from build123d import *

# Parameters (mm, degrees)
SKETCH3_R               = 2
SKETCH3_R_2             = 2.5
BOSS_EXTRUDE3_DEPTH     = 10
SKETCH4_W               = 29.621982307
SKETCH4_H               = 15
SKETCH4_W_2             = 29.629902686
BOSS_EXTRUDE4_DEPTH     = 15
FILLET1_R               = 10
CUT_EXTRUDE1_DEPTH      = 57
CUT_EXTRUDE1_DEPTH_BACK = 15
SKETCH5_R               = 4
FILLET3_R               = 10


with BuildPart() as part:
    # Sketch3 → Boss-Extrude3 (new body)
    with BuildSketch(Plane(origin=(0, 0, 0), x_dir=(1, 0, 0), z_dir=(0, 1, 0))):
        with BuildLine():
            Line((-74.553080605, -18.028525235), (-74.553080605, 16.971474765))
            Line((-74.553080605, 16.971474765), (75.446919395, 16.971474765))
            Line((75.446919395, 16.971474765), (75.446919395, -18.028525235))
            Line((75.446919395, -18.028525235), (75.446919395, -59.351917417))
            ThreePointArc((75.446919395, -59.351917417), (72.517987207, -66.422985229), (65.446919395, -69.351917417))
            Line((65.446919395, -69.351917417), (49.960719272, -69.351917417))
            ThreePointArc((49.960719272, -69.351917417), (47.125982353, -68.941717551), (44.523807175, -67.744770737))
            Line((44.523807175, -67.744770737), (5.883831491, -42.713694512))
            ThreePointArc((5.883831491, -42.713694512), (0.446919395, -41.106547832), (-4.989992702, -42.713694512))
            Line((-4.989992702, -42.713694512), (-43.629968386, -67.744770737))
            ThreePointArc((-43.629968386, -67.744770737), (-46.232143563, -68.941717551), (-49.066880482, -69.351917417))
            Line((-49.066880482, -69.351917417), (-64.553080605, -69.351917417))
            ThreePointArc((-64.553080605, -69.351917417), (-71.624148417, -66.422985229), (-74.553080605, -59.351917417))
            Line((-74.553080605, -59.351917417), (-74.553080605, -18.028525235))
        make_face()
        with Locations(Location((-68.553080605, 11.471474765, 0), (0, 0, 270))):
            Circle(SKETCH3_R, mode=Mode.SUBTRACT)
        with Locations(Location((-50.553080605, 11.471474765, 0), (0, 0, 270))):
            Circle(SKETCH3_R, mode=Mode.SUBTRACT)
        with Locations(Location((-68.553080605, -12.528525235, 0), (0, 0, 270))):
            Circle(SKETCH3_R, mode=Mode.SUBTRACT)
        with Locations(Location((-50.553080605, -12.528525235, 0), (0, 0, 270))):
            Circle(SKETCH3_R, mode=Mode.SUBTRACT)
        with Locations(Location((51.446919395, -12.528525235, 0), (0, 0, 90))):
            Circle(SKETCH3_R, mode=Mode.SUBTRACT)
        with Locations(Location((69.446919395, -12.528525235, 0), (0, 0, 90))):
            Circle(SKETCH3_R, mode=Mode.SUBTRACT)
        with Locations(Location((69.446919395, 11.471474765, 0), (0, 0, 90))):
            Circle(SKETCH3_R, mode=Mode.SUBTRACT)
        with Locations(Location((51.446919395, 11.471474765, 0), (0, 0, 90))):
            Circle(SKETCH3_R, mode=Mode.SUBTRACT)
        with Locations(Location((-50.553080605, -47.693315976, 0), (0, 0, 270))):
            Circle(SKETCH3_R_2, mode=Mode.SUBTRACT)
        with Locations(Location((51.446919395, -47.693315976, 0), (0, 0, 90))):
            Circle(SKETCH3_R_2, mode=Mode.SUBTRACT)
    extrude(amount=BOSS_EXTRUDE3_DEPTH)

    # Sketch4 → Boss-Extrude4 (add)
    with BuildSketch(Plane.XZ):
        with Locations((-59.742089452, 0)):
            Rectangle(SKETCH4_W, SKETCH4_H)
        with Locations((60.624047673, 0)):
            Rectangle(SKETCH4_W_2, SKETCH4_H)
        with Locations((60.624047673, 51.713197214)):
            Rectangle(SKETCH4_W_2, SKETCH4_H)
        with Locations((-59.742089452, 51.713197214)):
            Rectangle(SKETCH4_W, SKETCH4_H)
    extrude(amount=BOSS_EXTRUDE4_DEPTH)

    # Fillet1
    fillet1_edges = [part.edges().sort_by_distance(p)[0] for p in [
        (-44.931098298, -15, 0),
        (-74.553080605, -15, 0),
        (75.438999016, -15, 0),
        (45.80909633, -15, 0),
    ]]
    fillet(fillet1_edges, radius=FILLET1_R)

    # Sketch5 → Cut-Extrude1 (cut, two sides: drawn at the far end of the back side and taken through both)
    with BuildSketch(Plane.XY.offset(7.5).offset(-CUT_EXTRUDE1_DEPTH_BACK)):
        with Locations(Location((-59.742089451, -7.004049179, 0), (0, 0, 180))):
            Circle(SKETCH5_R)
        with Locations(Location((60.620087484, -7.004049179, 0), (0, 0, 180))):
            Circle(SKETCH5_R)
    extrude(amount=CUT_EXTRUDE1_DEPTH + CUT_EXTRUDE1_DEPTH_BACK, mode=Mode.SUBTRACT)

    # Fillet3
    fillet3_edges = [part.edges().sort_by_distance(p)[0] for p in [
        (45.80909633, -15, 51.713197214),
        (75.438999016, -15, 51.713197214),
        (-74.553080605, -15, 51.713197214),
        (-44.931098298, -15, 51.713197214),
    ]]
    fillet(fillet3_edges, radius=FILLET3_R)


solid = part.part
For this review, take the finished solid that the model builds, in its own axes (mm). A direction names the side the tool comes from. Round coordinates to 2 decimals unless told otherwise and drop trailing zeros. Loops run counter-clockwise (first coordinate to the right, second up) from the corner with the lowest first, then second, coordinate; pieces in that order, holes last. Notation, with made-up numbers: (40.25, 8.5) - (59.25, 8.5) arc R29 cw to (59.25, 29.5) - close; hole circle Ø4 at (-25.75, 23). An arc over 180 degrees is marked (long way). Use one line per item in the form item = value.
1) Wall thickness on probe 1 along X at (y, z) = (-2.5, 50); probe 2 along Z at (x, y) = (48, -4); probe 3 along Z at (x, y) = (-67, 6.5): over which ranges is each line inside the solid? List them lowest first.
Solutions:
probe_1 = -74.55 to -44.93, 45.81 to 75.44
probe_2 = -7.5 to 7.5, 44.21 to 59.21
probe_3 = -16.97 to -12.73, -10.21 to 11.27, 13.79 to 69.05
2) Clearance check with flat-ended pins moving along their axes: P1, Ø7.5, axis at x = -59.5, y = -9.5, coming from the -Z side; P2, Ø2.5, axis at y = -3, z = -1.5, coming from the +X side; P3, Ø4.5, axis at x = -68.55, z = 12.53, coming from the -Y side; P4, Ø3.5, axis at x = -50.55, z = -11.47, coming from the -Y side. State where each tip first meets the part, or that it passes through.
Solutions:
P1 = -7.5
P2 = 75.44
P3 = 0
P4 = through
3) Mouldability with a two-part tool opening along Z and no side actions: class faces 1 (the face through (-24.04, 4.93, 55.054)), 2 (the face through (64, -4, 7.5)), 3 (the face through (75.439, -2, 52)), 4 (the face through (53.221, 4.93, 11.606)) as pulls with the +Z half, pulls with the -Z half, needs draft (parallel to the pull), parting line crosses it, or undercut.
Solutions:
face_1 = pulls with the +Z half
face_2 = undercut
face_3 = needs draft
face_4 = undercut
4) We need section B-B on x = 58.5. Write out the cut boundary in (y, z), then the cut area to 3 significant figures.
Solutions:
outline = (-15, -7.5) - (-10.4, -7.5) - (-10.4, 7.5) - (-15, 7.5) - close; (-15, 44.21) - (-10.4, 44.21) - (-10.4, 59.21) - (-15, 59.21) - close; (-3.61, -7.5) - (0, -7.5) - (0, -16.97) - (10, -16.97) - (10, 69.35) - (0, 69.35) - (0, 59.21) - (-3.61, 59.21) - (-3.61, 44.21) - (0, 44.21) - (0, 7.5) - (-3.61, 7.5) - close
area = 1,110 mm2
5) Tool access review of faces 5 (the face through (-51.511, 4.93, 50.003)), 6 (the face through (-56.7, -4.1, -7.5)), 7 (the face through (25.47, 4.93, 55.4)), 8 (the face through (45.809, -2, 52)): name each direction out of +Z, -Z, +X, -X, +Y, -Y from which nothing blocks a thin tool from reaching the whole face with its end or side.
Solutions:
face_5 = +Y
face_6 = -Z, +X, -X, -Y
face_7 = +Z, +Y, -Y
face_8 = +Z, -Z, -Y
6) We need section A-A on z = 54. State how many separate pieces and enclosed holes the cut face has, then the cut area to 3 significant figures.
Solutions:
separate_pieces = 2
enclosed_holes = 2
area = 1,750 mm2
